Autodesk Inventor part; units mm, degrees
ref_plane "YZ Plane" through (0, 0, 0) normal (1, 0, 0) x (0, 1, 0)
ref_plane "XZ Plane" through (0, 0, 0) normal (0, 1, 0) x (-1, 0, 0)
ref_plane "XY Plane" through (0, 0, 0) normal (0, 0, 1) x (1, 0, 0)
sketch "Sketch1" plane through (0, 0, 0) normal (0, 0, 1) x (1, 0, 0)
  line L0 (0, 0) -> (352.425, 0)
  line L1 (352.425, 0) -> (352.425, 114.3)
  line L2 (352.425, 114.3) -> (0, 114.3)
  line L3 (0, 114.3) -> (0, 0)
  dimension "d0" = 352.425
  dimension "d1" = 114.3
extrude "Extrusion1" add sketch "Sketch1" along normal blind 3.175
sketch "Sketch2" plane through (0, 0, 3.175) normal (0, 0, 1) x (1, 0, 0)
  line L0 (12.7, 0) -> (339.725, 0)
  line L1 (339.725, 0) -> (339.725, 38.1)
  line L2 (339.725, 38.1) -> (12.7, 38.1)
  line L3 (12.7, 38.1) -> (12.7, 0)
  line L4 (0, 114.3) -> (0, 0)
  line L5 (352.425, 0) -> (352.425, 114.3)
  dimension "d4" = 12.7
  dimension "d5" = 12.7
  dimension "d6" = 38.1
extrude "Extrusion2" cut sketch "Sketch2" against normal blind 25.4
sketch "Sketch3" plane through (0, 0, 3.175) normal (0, 0, 1) x (1, 0, 0)
  line L0 (339.725, 38.1) -> (12.7, 38.1)
  line L1 (85.09, 38.1) -> (129.54, 38.1)
  line L2 (129.54, 38.1) -> (129.54, 101.6)
  line L3 (129.54, 101.6) -> (85.09, 101.6)
  line L4 (85.09, 101.6) -> (85.09, 38.1)
  point P0 (0, 0)
  dimension "d9" = 63.5
  dimension "d10" = 72.39
  dimension "d11" = 44.45
extrude "Extrusion3" cut sketch "Sketch3" against normal blind 25.4
properties part number "SmallWall"
Design review of the part built by this model. Coordinates are the model's own, in mm. Round coordinates to 2 decimals unless told otherwise and drop trailing zeros. Loops run counter-clockwise (first coordinate to the right, second up) from the corner with the lowest first, then second, coordinate; pieces in that order, holes last. Notation, with made-up numbers: (-6, 26) - (-2, 26) arc R24 ccw to (-2, 55) - close; hole circle Ø7 at (9, 75.5). An arc over 180 degrees is marked (long way). One line per item, written item: value. Start each with the question number.
1) Consider section C-C on y = 17. Give the boundary of the cut face in (x, z) (3 decimals), then the cut area to 3 significant figures.
2) Insertion check: pin 1 Ø1.5 at (x, z) = (86, 2.5) entering from -Y. The pin has a flat end and moves straight along its axis. Give the tip position at first contact, or say it passes through.
3) Consider section B-B on z = 1.55. Give the boundary of the cut face in (x, y) (3 decimals), then the cut area to 3 significant figures.
4) Consider section D-D on x = 196. Give the boundary of the cut face in (y, z) (3 decimals).
5) To check wall thickness, follow L1, parallel to X at y = 13, z = 0.5 (3 decimals); L2, parallel to X at y = 80, z = 0.5 (3 decimals); L3, parallel to Y at x = 228, z = 1.8. State the ranges of each line that lie inside material, in increasing order. Write a range as from..to.
6) Consider section A-A on y = 81. Give the boundary of the cut face in (x, z) (3 decimals).
Reported:
1. outline: (0, 0) - (12.7, 0) - (12.7, 3.175) - (0, 3.175) - close; (339.725, 0) - (352.425, 0) - (352.425, 3.175) - (339.725, 3.175) - close
1. area: 80.6 mm^2
2. pin 1: stops at y = 101.6
3. outline: (0, 0) - (12.7, 0) - (12.7, 38.1) - (85.09, 38.1) - (85.09, 101.6) - (129.54, 101.6) - (129.54, 38.1) - (339.725, 38.1) - (339.725, 0) - (352.425, 0) - (352.425, 114.3) - (0, 114.3) - close
3. area: 25,000 mm^2
4. outline: (38.1, 0) - (114.3, 0) - (114.3, 3.175) - (38.1, 3.175) - close
5. L1: x = 0..12.7, 339.725..352.425
5. L2: x = 0..85.09, 129.54..352.425
5. L3: y = 38.1..114.3
6. outline: (0, 0) - (85.09, 0) - (85.09, 3.175) - (0, 3.175) - close; (129.54, 0) - (352.425, 0) - (352.425, 3.175) - (129.54, 3.175) - close
